Geometry check sheet. Reference: drawing and pictorial views, mm from the part's lowest x, y, z. A direction names the side the tool comes from. Give positions to 0.01 mm unless a question says otherwise; leave off trailing zeros. Write each loop counter-clockwise with the first axis right and the second up, starting at its lowest first coordinate (ties: lowest second). Pieces come first, ordered by that corner, then holes. Notation, with made-up numbers: M 39,9.5 L 74,9.5 A11 ccw 74,24.5 Z; hole C -6.75,18 d5. An arc over 180 degrees is marked long. Write item = value, one per line. Start each with the question number.
1) Cross-section at C-C, the plane z = 19. Record the cut outline in (x, y) (1 decimal).
2) Scan lines: line 1 along X through (y, z) = (10, 16) (1 decimal); line 2 along Z through (x, y) = (21, 12); line 3 along X through (y, z) = (6.25, 49.5) (1 decimal). Record each from-to range of solid material in increasing order. Write a range as [from, to].
3) Cross-section at D-D, the plane x = 117.5. Record the cut outline in (y, z), plus the area to 3 significant figures.
4) Mould release check, pull along X, two halves, no side actions. Record for the marked faces 1, 2 and 3: released by +X, released by -X, zero draft, split by the parting line, or undercut.
5) Access from +Z, -Z, +X, -X, +Y, -Y to the whole of each face (thin tool, end or side, straight path). Record for the marked faces 4, 5 and 6.
6) Go/stop test with flat-tipped pins: pin 1 (15 mm diameter, centred on x = 13.5, y = 15, fed in from +Z); pin 2 (14.5 mm diameter, centred on y = 10, z = 120.5, fed in from +X); pin 3 (6 mm diameter, centred on x = 20, y = 9.5, fed in from -Z). Record where each tip stops, or that it passes through.
7) Cross-section at A-A, the plane z = 60.5. Record the cut outline in (x, y) (1 decimal), plus the area to 3 significant figures.
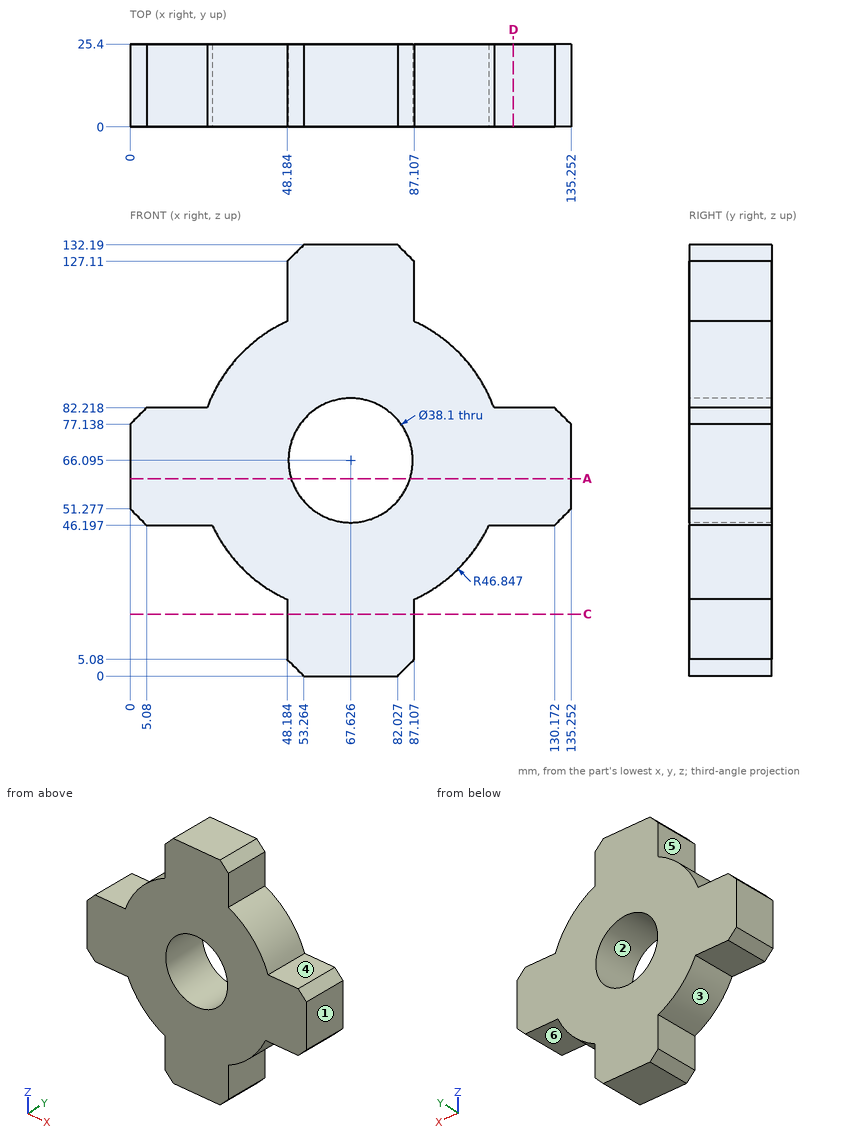
Reply:
q1.outline = M 48.2,0 L 87.1,0 L 87.1,25.4 L 48.2,25.4 Z
q2.line_1 = [48.2, 87.1]
q2.line_2 = [46.2, 82.22]
q2.line_3 = [1.8, 58.3], [77, 133.5]
q3.outline = M 0,46.2 L 25.4,46.2 L 25.4,82.22 L 0,82.22 Z
q3.area = 915 mm2
q4.face_1 = released by +X
q4.face_2 = undercut
q4.face_3 = released by -X
q5.face_4 = +Z, +X, +Y, -Y
q5.face_5 = +Z, -X, +Y, -Y
q5.face_6 = -Z, +X, +Y, -Y
q6.pin_1 = 82.22
q6.pin_2 = 87.11
q6.pin_3 = 46.2
q7.outline = M 0,0 L 49.4,0 L 49.4,25.4 L 0,25.4 Z; M 85.8,0 L 135.3,0 L 135.3,25.4 L 85.8,25.4 Z
q7.area = 2,510 mm2
